from build123d import *

# Parameters (mm, degrees)
F1_DEPTH = 63.5
F0_W     = 25.7323723912
F0_H     = 19.05
F2_DEPTH = 25.4
F3_DEPTH = 25.4
F4_DEPTH = 7.9375
F6_R     = 5.08


with BuildPart() as f1:
    # F0 (on Front) → F1 (new body, symmetric)
    with BuildSketch(Plane.XZ):
        Polygon((22.225, 9.525), (-41.275, 9.525), (-41.275, -9.525), (41.275, -9.525), (41.275, 9.525), align=None)
    extrude(amount=F1_DEPTH, both=True)

    # F0 (on Front) → F2 (join, symmetric)
    with BuildSketch(Plane.XZ):
        with BuildLine():
            Line((22.225, 46.0502), (22.225, 9.525))
            Line((22.225, 9.525), (41.275, 9.525))
            Line((41.275, 9.525), (41.275, 46.0502))
            ThreePointArc((41.275, 46.0502), (45.9246798487, 57.2755201513), (57.15, 61.9252))
            Line((57.15, 61.9252), (60.325, 61.9252))
            Line((60.325, 61.9252), (60.325, 80.9752))
            Line((60.325, 80.9752), (57.15, 80.9752))
            add(Edge.make_bspline(
                [(56.2643970704, 80.9639699547), (56.5604917652, 80.9691161727), (56.8557023266, 80.972860747), (57.15, 80.9752)],
                knots=[120.7425968685, 120.7425968685, 120.7425968685, 120.7425968685, 121.6248811101, 121.6248811101, 121.6248811101, 121.6248811101], degree=3))
            ThreePointArc((56.2643970704, 80.9639699547), (32.1431478659, 70.4307859516), (22.225, 46.0502))
        make_face()
        with Locations((73.1911861956, 71.4502)):
            Rectangle(F0_W, F0_H)
    extrude(amount=F2_DEPTH, both=True)

    # F0 (on Front) → F3 (join, symmetric)
    with BuildSketch(Plane.XZ):
        with BuildLine():
            Line((22.225, 46.0502), (22.225, 9.525))
            Line((22.225, 9.525), (41.275, 9.525))
            Line((41.275, 9.525), (41.275, 46.0502))
            ThreePointArc((41.275, 46.0502), (45.9246798487, 57.2755201513), (57.15, 61.9252))
            Line((57.15, 61.9252), (60.325, 61.9252))
            Line((60.325, 61.9252), (60.325, 80.9752))
            Line((60.325, 80.9752), (57.15, 80.9752))
            add(Edge.make_bspline(
                [(56.2643970704, 80.9639699547), (56.5604917652, 80.9691161727), (56.8557023266, 80.972860747), (57.15, 80.9752)],
                knots=[120.7425968685, 120.7425968685, 120.7425968685, 120.7425968685, 121.6248811101, 121.6248811101, 121.6248811101, 121.6248811101], degree=3))
            ThreePointArc((56.2643970704, 80.9639699547), (32.1431478659, 70.4307859516), (22.225, 46.0502))
        make_face()
        with Locations((73.1911861956, 71.4502)):
            Rectangle(F0_W, F0_H)
    extrude(amount=F3_DEPTH, both=True)

    # F0 (on Front) → F4 (join, symmetric)
    with BuildSketch(Plane.XZ):
        with BuildLine():
            add(Edge.make_bspline(
                [(-41.275, 9.525), (-41.3365892796, 53.3046842853), (15.7431674311, 80.2596983695), (56.2643970704, 80.9639699547)],
                knots=[0, 0, 0, 0, 120.7425968685, 120.7425968685, 120.7425968685, 120.7425968685], degree=3))
            Line((-41.275, 9.525), (22.225, 9.525))
            Line((22.225, 9.525), (22.225, 46.0502))
            ThreePointArc((22.225, 46.0502), (32.1431478659, 70.4307859516), (56.2643970704, 80.9639699547))
        make_face()
    extrude(amount=F4_DEPTH, both=True)

    # F0 (on Front) → F5 (revolve)
    with BuildSketch(Plane.XZ):
        Polygon((86.0573723912, 85.725), (86.0573723912, 80.9752), (86.0573723912, 61.9252), (86.0573723912, 57.15), (111.125, 57.15), (111.125, 85.725), align=None)
    revolve(axis=Axis((86.0573723912, 0, 71.4375), (0, 0, -1)))

    # F6
    f6_edges = [f1.edges().sort_by_distance(p)[0] for p in [
        (-41.275, 63.5, 0),
        (-41.275, -63.5, 0),
        (41.275, 63.5, 0),
        (41.275, -63.5, 0),
    ]]
    fillet(f6_edges, radius=F6_R)


solid = f1.part
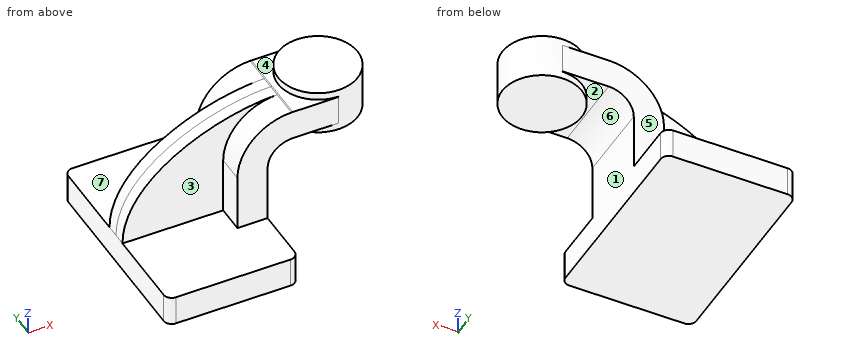
Source: CAD feature listing. Evaluate the final solid. Frame: model axes, mm. Face numbers are marked on the shaded views. A direction names the side the tool comes from. Round coordinates to 2 decimals unless told otherwise and drop trailing zeros. Write each loop counter-clockwise with the first axis right and the second up, starting at its lowest first coordinate (ties: lowest second). Pieces come first, ordered by that corner, then holes. Notation, with made-up numbers: M 21,52.5 L 70,52.5 A25 cw 70,84.5 Z; hole C -29.5,50 d4. An arc over 180 degrees is marked long. One line per item, written item: value. Start each with the question number.
Item 1: Pin query (flat end, axial travel): pin 1 (2 mm diameter, centred on x = 4.5, z = 64, fed in from -Y); pin 2 (1 mm diameter, centred on x = -5, y = 34.5, fed in from +Z) (3 decimals); pin 3 (14 mm diameter, centred on y = -19, z = 34, fed in from -X) (3 decimals). Return the tip coordinate at first contact, or that it passes through.
Item 2: Ray query, L1, parallel to Y at x = -12, z = 30.5; L2, parallel to Z at x = 99, y = -13 (3 decimals); L3, parallel to Z at x = -4, y = 15.5 (3 decimals). Return the intervals inside material, ascending. Write a range as from..to.
Item 3: Set-up query: the marked faces 4, 5, 6 and 7. Return all of +Z, -Z, +X, -X, +Y, -Y with unobstructed straight access to the full face (end or side cutting, diameter ignored); none if empty.
Item 4: Mould query, pull axis X, two halves, no side actions, for the marked faces 1, 2 and 3. Classes: pulls with the +X half, pulls with the -X half, needs draft (parallel to the pull), parting line crosses it, or undercut.
Item 5: Section query B-B (y = -29.5). Return the cut outline in (x, z) (3 decimals), plus the area to 3 significant figures.
Item 6: Section query A-A (z = 1). Return the cut outline in (x, y) (3 decimals), plus the area to 3 significant figures.
Result set:
1. pin 1: stops at y = -7.94
1. pin 2: stops at z = 9.525
1. pin 3: stops at x = 22.225
2. L1: y = -7.94..7.94
2. L2: z = 57.15..85.725
2. L3: z = -9.525..9.525
3. face 4: +Z, -X
3. face 5: +Z, +X, -X, +Y
3. face 6: -Z, +Y, -Y
3. face 7: +Z, -X, +Y
4. face 1: pulls with the +X half
4. face 2: undercut
4. face 3: needs draft
5. outline: M -41.275,-9.525 L 41.275,-9.525 L 41.275,9.525 L -41.275,9.525 Z
5. area: 1,570 mm²
6. outline: M -41.275,-58.42 A5.08 ccw -36.195,-63.5 L 36.195,-63.5 A5.08 ccw 41.275,-58.42 L 41.275,58.42 A5.08 ccw 36.195,63.5 L -36.195,63.5 A5.08 ccw -41.275,58.42 Z
6. area: 10,500 mm²
